Input: part model. Units: mm. Frame: model coordinates. Coordinates: 2 decimals unless noted, no trailing zeros. Order: outer loops, then holes, each group sorted by start corner. A loop starts at its lowest first (then second) coordinate and runs counter-clockwise, first axis right, second up. Notation, with made-up numbers: (5, -1.5) -> (33, -1.5) arc R26 cw to (33, 28.5) -> close; hole circle Ø4 at (-23, 12). An arc over 180 degrees is marked (long way). Answer as CSV lines item,"result".
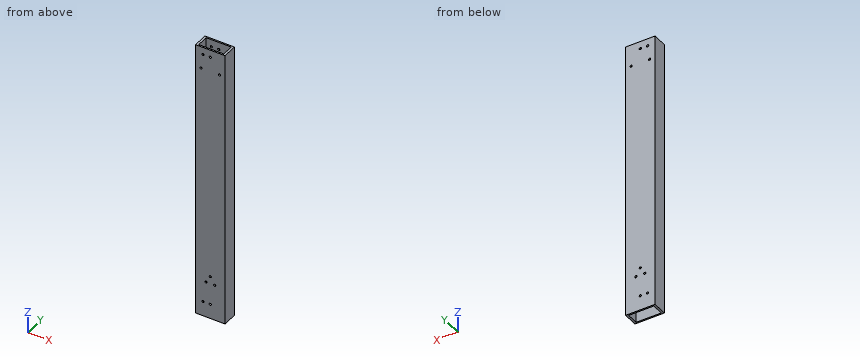
Solid Edge part; units mm, degrees
sketch "Sketch1" plane through (0, 0, 0) normal (0, 0, 1) x (1, 0, 0)
  line L0 (-17, -8) -> (17, -8)
  line L1 (17, -8) -> (17, 8)
  line L2 (17, 8) -> (-17, 8)
  line L3 (-17, 8) -> (-17, -8)
  line L4 (-20, -10) -> (20, -10)
  line L5 (20, -10) -> (20, 10)
  line L6 (20, 10) -> (-20, 10)
  line L7 (-20, 10) -> (-20, -10)
  dimension "D1" = 20
  dimension "D2" = 20
  dimension "D3" = 20
  dimension "D4" = 17
  dimension "D5" = 17
extrude "Protrusion1" add sketch "Sketch1" along normal blind 500
sketch "Sketch2" plane through (0, 0, 0) normal (0, -1, 0) x (1, 0, 0)
  circle A0 centre (-6, 49.2) radius 1.5
  circle A1 centre (6, 49.2) radius 1.5
  circle A2 centre (0, 59.2) radius 1.5
extrude "ExtrudedCutout_1" cut sketch "Sketch2" along normal mid plane 184.7179
sketch "Sketch3" plane through (0, -10, 250) normal (0, -1, 0) x (0, 0, 1)
  circle A0 centre (-230, 10) radius 1.5
  circle A1 centre (-230, 0) radius 1.5
  dimension "D1" = 230
extrude "VaciadoExtruido_2" cut sketch "Sketch3" against normal blind 109.5957
sketch "Sketch4" plane through (0, -10, 250) normal (0, -1, 0) x (0, 0, 1)
  circle A0 centre (99.2, 12.5) radius 1.5
  circle A1 centre (99.2, -12.5) radius 1.5
extrude "VaciadoExtruido_3" cut sketch "Sketch4" along normal mid plane 772.9551
sketch "Sketch5" plane through (20, 0, 250) normal (1, 0, 0) x (0, 0, 1)
  line L0 (129.2, 28.1693) -> (129.2, -48.5485)
  line L1 (267.5229, -23.3945) -> (129.2, -48.5485)
  line L2 (267.5229, 33.3028) -> (267.5229, -23.3945)
  line L3 (129.2, 28.1693) -> (267.5229, 33.3028)
extrude "VaciadoExtruido_4" cut sketch "Sketch5" along normal mid plane 530
sketch "Sketch6" plane through (0, -10, 189.6) normal (0, -1, 0) x (0, 0, 1)
  circle A0 centre (179.6, 10) radius 1.5
  circle A1 centre (179.6, 0) radius 1.5
extrude "VaciadoExtruido_5" cut sketch "Sketch6" along normal mid plane 1696
1. Ray query, line 1 along X through (y, z) = (8.55, 369.2); line 2 along X through (y, z) = (-9.3, 349.2); line 3 along Y through (x, z) = (5.5, 219). Return the intervals inside material, ascending.
Findings:
line 1,"x = -20 to -11.5, -8.5 to -1.5, 1.5 to 20"
line 2,"x = -20 to -14, -11 to 11, 14 to 20"
line 3,"y = -10 to -8, 8 to 10"
2. Contact query for flat-ended pins moving along their axis: pin 1 (5 mm diameter, centred on x = -6, z = 49.2, fed in from +Y); pin 2 (2.5 mm diameter, centred on x = 12.5, z = 349.2, fed in from +Y). Output: stop coordinate, or through.
Findings:
pin 1,"stops at y = 10"
pin 2,"passes through"
3. Cut plane B-B (z = 186). Return the cut outline in (x, y).
Findings:
outline,"(-20, -10) -> (20, -10) -> (20, 10) -> (-20, 10) -> close; hole (-17, -8) -> (17, -8) -> (17, 8) -> (-17, 8) -> close"
4. Cut plane A-A (y = 0.5). Return the cut outline in (x, z), plus the area to 3 significant figures.
Findings:
outline,"(-20, 0) -> (-17, 0) -> (-17, 379.2) -> (-20, 379.2) -> close; (17, 0) -> (20, 0) -> (20, 379.2) -> (17, 379.2) -> close"
area,"2,280 mm2"
